Work out the finished part from the listing and answer in its coordinate system (mm). Face numbers are marked on the shaded views. A direction names the side the tool comes from. Give positions to 0.01 mm unless a question says otherwise; leave off trailing zeros. Loops run counter-clockwise (first coordinate to the right, second up) from the corner with the lowest first, then second, coordinate; pieces in that order, holes last. Notation, with made-up numbers: M -3.5,-6.75 L 5.5,-6.75 A23 cw 5.5,24.25 Z; hole C 11,-20.5 d10. An arc over 180 degrees is marked long. Use a Markdown table: item, result.
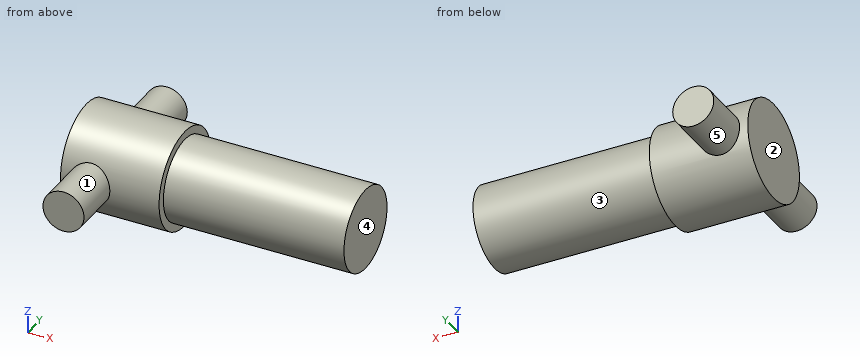
```python
from build123d import *

# Parameters (mm, degrees)
F0_R     = 3
F1_DEPTH = 6
F2_R     = 2.5
F3_DEPTH = 11
F4_R     = 1.25
F5_DEPTH = 6


with BuildPart() as f1:
    # F0 (on Right) → F1 (new body)
    with BuildSketch(Plane.YZ):
        Circle(F0_R)
    extrude(amount=F1_DEPTH)

    # F2 (on face) → F3 (join)
    with BuildSketch(Plane.YZ.offset(6)):
        Circle(F2_R)
    extrude(amount=F3_DEPTH)

    # F4 (on Front) → F5 (join, symmetric)
    with BuildSketch(Plane.XZ):
        with Locations((1.75, 0)):
            Circle(F4_R)
    extrude(amount=F5_DEPTH, both=True)


solid = f1.part
```
(1) Consider probe 1 along X at (y, z) = (-1.25, 2.5); probe 2 along Z at (x, y) = (12, -1.25); probe 3 along X at (y, z) = (3, 1). Determine where each line is inside the solid, lowest interval first. Write a range as [from, to].
Entries:
| item | result |
|---|---|
| probe 1 | x = [0, 6] |
| probe 2 | z = [-2.17, 2.17] |
| probe 3 | x = [1, 2.5] |
(2) A cutting plane is placed at C-C (x = 1.75). Write down the section's boundary in (y, z).
Entries:
| item | result |
|---|---|
| outline | M -6,-1.25 L -2.73,-1.25 A3 ccw 2.73,-1.25 L 6,-1.25 L 6,1.25 L 2.73,1.25 A3 ccw -2.73,1.25 L -6,1.25 Z |
(3) Which of the six approach directions +Z, -Z, +X, -X, +Y, -Y give full straight-line access (tool end or side, diameter ignored) to the marked faces 1, 2, 3, 4 and 5?
Entries:
| item | result |
|---|---|
| face 1 | -Y |
| face 2 | +Z, -Z, -X, +Y, -Y |
| face 3 | +X |
| face 4 | +Z, -Z, +X, +Y, -Y |
| face 5 | +Y |
(4) A cutting plane is placed at B-B (z = 0). Write down the section's boundary in (x, y), and give its area (3 significant figures).
Entries:
| item | result |
|---|---|
| outline | M 0,-3 L 0.5,-3 L 0.5,-6 L 3,-6 L 3,-3 L 6,-3 L 6,-2.5 L 17,-2.5 L 17,2.5 L 6,2.5 L 6,3 L 3,3 L 3,6 L 0.5,6 L 0.5,3 L 0,3 Z |
| area | 106 mm² |
(5) A cutting plane is placed at D-D (x = 6.5). Write down the section's boundary in (y, z), and give its area (3 significant figures).
Entries:
| item | result |
|---|---|
| outline | C 0,0 d5 |
| area | 19.6 mm² |
(6) A cutting plane is placed at A-A (y = 0). Write down the section's boundary in (x, z), and give its area (3 significant figures).
Entries:
| item | result |
|---|---|
| outline | M 0,-3 L 6,-3 L 6,-2.5 L 17,-2.5 L 17,2.5 L 6,2.5 L 6,3 L 0,3 Z |
| area | 91.0 mm² |
(7) Given P1, Ø1, axis at x = 10, y = -2.5, coming from the -Z side; P2, Ø2, axis at y = 4.5, z = -1, coming from the +X side; P3, Ø1, axis at x = 9.5, y = -1.5, coming from the -Z side, each flat-ended and moving along its own axis, determine where each tip first touches the part or whether it passes through.
Entries:
| item | result |
|---|---|
| P1 | stops at z = -1.5 |
| P2 | stops at x = 3 |
| P3 | stops at z = -2.29 |
